Verification items for the finished model (mm, model axes). Face numbers are marked on the shaded views. Round coordinates to 2 decimals unless told otherwise and drop trailing zeros. Write each loop counter-clockwise with the first axis right and the second up, starting at its lowest first coordinate (ties: lowest second). Pieces come first, ordered by that corner, then holes. Notation, with made-up numbers: (3, -2) -> (31, -2) arc R12 cw to (31, 19) -> close; hole circle Ø8 at (66.25, 65). An arc over 180 degrees is marked (long way). Answer as a JSON object with one key per item and string values. Group by question number.
(1) Sectioned sample at A-A on x = 117.5. Record the cut outline in (y, z).
(2) Scan lines: L1, parallel to Y at x = 65, z = 8.55; L2, parallel to X at y = 44, z = 9.25; L3, parallel to Y at x = 113.5, z = 6.75. Record each from-to range of solid material in increasing order. Write a range as from..to.
(3) Gauge pin test, flat ends, axial feed: pin 1 Ø12 at (x, y) = (67, 18) entering from +Z; pin 2 Ø1.5 at (x, y) = (100.5, 12) entering from +Z. Record the tip position at first contact, or that the pin passes through.
(4) Draft check along Y on the marked faces 1, 2 and 3. Enter one of: released by +Y, released by -Y, zero draft, split by the parting line, or undercut.
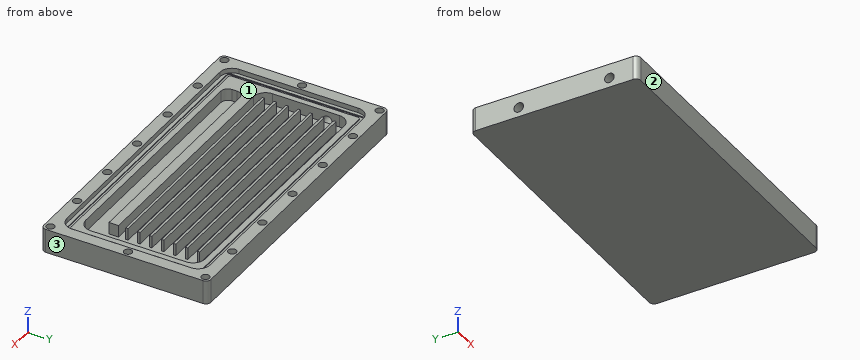
```python
from build123d import *

# Parameters (mm, degrees)
BOSS_EXTRU_1_DEPTH      = 10
ENL_V_MAT_EXTRU_1_DEPTH = 2
ENL_V_MAT_EXTRU_3_DEPTH = 5
ESQUISSE23_W            = 98
ESQUISSE23_H            = 1
BOSS_EXTRU_2_DEPTH      = 5
ENL_V_MAT_EXTRU_4_DEPTH = 0.4
ESQUISSE19_R            = 2
ENL_V_MAT_EXTRU_5_DEPTH = 10
D_GAGEMENT_M31_D        = 3.4
D_GAGEMENT_M31_DEPTH    = 3.978536948
D_GAGEMENT_M31_TIP      = 1.021463052


with BuildPart() as part:
    # Esquisse1 → Boss.-Extru.1 (new body)
    with BuildSketch(Plane.XY):
        with BuildLine():
            Line((2, 0), (128, 0))
            ThreePointArc((128, 0), (129.414213562, 0.585786438), (130, 2))
            Line((130, 2), (130, 68))
            ThreePointArc((130, 68), (129.414213562, 69.414213562), (128, 70))
            Line((128, 70), (2, 70))
            ThreePointArc((2, 70), (0.585786438, 69.414213562), (0, 68))
            Line((0, 68), (0, 2))
            ThreePointArc((0, 2), (0.585786438, 0.585786438), (2, 0))
        make_face()
    extrude(amount=BOSS_EXTRU_1_DEPTH)

    # Esquisse18 → Enlèv. mat.-Extru.1 (cut)
    with BuildSketch(Plane.XY.offset(10)):
        with BuildLine():
            Line((10, 5), (120, 5))
            ThreePointArc((120, 5), (123.535533906, 6.464466094), (125, 10))
            Line((125, 10), (125, 60))
            ThreePointArc((125, 60), (123.535533906, 63.535533906), (120, 65))
            Line((120, 65), (10, 65))
            ThreePointArc((10, 65), (6.464466094, 63.535533906), (5, 60))
            Line((5, 60), (5, 10))
            ThreePointArc((5, 10), (6.464466094, 6.464466094), (10, 5))
        make_face()
    extrude(amount=-ENL_V_MAT_EXTRU_1_DEPTH, mode=Mode.SUBTRACT)

    # Esquisse20 → Enlèv. mat.-Extru.3 (cut)
    with BuildSketch(Plane.XY.offset(8)):
        with BuildLine():
            Line((15, 60), (115, 60))
            ThreePointArc((115, 60), (118.535533906, 58.535533906), (120, 55))
            Line((120, 55), (120, 15))
            ThreePointArc((120, 15), (118.535533906, 11.464466094), (115, 10))
            Line((115, 10), (18, 10))
            ThreePointArc((18, 10), (15.878679656, 10.878679656), (15, 13))
            Line((15, 13), (15, 15))
            ThreePointArc((15, 15), (15.878679656, 17.121320344), (18, 18))
            Line((18, 18), (112, 18))
            Line((112, 18), (112, 22))
            Line((112, 22), (15, 22))
            ThreePointArc((15, 22), (11.464466094, 23.464466094), (10, 27))
            Line((10, 27), (10, 55))
            ThreePointArc((10, 55), (11.464466094, 58.535533906), (15, 60))
        make_face()
    extrude(amount=-ENL_V_MAT_EXTRU_3_DEPTH, mode=Mode.SUBTRACT)

    # Esquisse23 → Boss.-Extru.2 (add)
    with BuildSketch(Plane.XY.offset(3)):
        with Locations((62.966066354, 55.5)):
            Rectangle(ESQUISSE23_W, ESQUISSE23_H)
        with Locations((62.966066354, 50.5)):
            Rectangle(ESQUISSE23_W, ESQUISSE23_H)
        with Locations((62.966066354, 45.5)):
            Rectangle(ESQUISSE23_W, ESQUISSE23_H)
        with Locations((62.966066354, 40.5)):
            Rectangle(ESQUISSE23_W, ESQUISSE23_H)
        with Locations((62.966066354, 35.5)):
            Rectangle(ESQUISSE23_W, ESQUISSE23_H)
        with Locations((62.966066354, 30.5)):
            Rectangle(ESQUISSE23_W, ESQUISSE23_H)
        with Locations((62.966066354, 25.5)):
            Rectangle(ESQUISSE23_W, ESQUISSE23_H)
    extrude(amount=BOSS_EXTRU_2_DEPTH)

    # Esquisse24 → Enlèv. mat.-Extru.4 (cut)
    with BuildSketch(Plane.XY.offset(8)):
        with BuildLine():
            Line((6.5, 62.5), (6.5, 7.5))
            ThreePointArc((6.5, 7.5), (6.792893219, 6.792893219), (7.5, 6.5))
            Line((7.5, 6.5), (7.967348912, 6.5))
            Line((7.967348912, 6.5), (122.5, 6.5))
            ThreePointArc((122.5, 6.5), (123.207106781, 6.792893219), (123.5, 7.5))
            Line((123.5, 7.5), (123.5, 62.5))
            ThreePointArc((123.5, 62.5), (123.207106781, 63.207106781), (122.5, 63.5))
            Line((122.5, 63.5), (7.5, 63.5))
            ThreePointArc((7.5, 63.5), (6.792893219, 63.207106781), (6.5, 62.5))
        make_face()
        with BuildLine():
            Line((8.6, 62.4), (121.4, 62.4))
            ThreePointArc((121.4, 62.4), (122.107106781, 62.107106781), (122.4, 61.4))
            Line((122.4, 61.4), (122.4, 8.6))
            ThreePointArc((122.4, 8.6), (122.107106781, 7.892893219), (121.4, 7.6))
            Line((121.4, 7.6), (8.6, 7.6))
            ThreePointArc((8.6, 7.6), (7.892893219, 7.892893219), (7.6, 8.6))
            Line((7.6, 8.6), (7.6, 61.4))
            ThreePointArc((7.6, 61.4), (7.892893219, 62.107106781), (8.6, 62.4))
        make_face(mode=Mode.SUBTRACT)
    extrude(amount=-ENL_V_MAT_EXTRU_4_DEPTH, mode=Mode.SUBTRACT)

    # Esquisse19 → Enlèv. mat.-Extru.5 (cut)
    with BuildSketch(Plane.ZY):
        with Locations((4, 50)):
            Circle(ESQUISSE19_R)
        with Locations((4, 12)):
            Circle(ESQUISSE19_R)
    extrude(amount=-ENL_V_MAT_EXTRU_5_DEPTH, mode=Mode.SUBTRACT)

    # Dégagement M31
    with Locations(Plane.XY.offset(10)):
        with Locations((127.5, 67.5), (108.32, 67.5), (86.66, 67.5), (65, 67.5), (43.34, 67.5), (21.68, 67.5), (2.5, 67.5), (2.5, 35), (2.5, 2.5), (21.68, 2.5), (43.34, 2.5), (65.266790711, 2.5), (86.66, 2.5), (108.32, 2.5), (127.5, 2.5), (127.5, 35)):
            Hole(D_GAGEMENT_M31_D / 2, depth=D_GAGEMENT_M31_DEPTH)
            with Locations((0, 0, -(D_GAGEMENT_M31_DEPTH + D_GAGEMENT_M31_TIP / 2))):  # 118° drill point
                Cone(0, D_GAGEMENT_M31_D / 2, D_GAGEMENT_M31_TIP, mode=Mode.SUBTRACT)


solid = part.part
```
Computed values:
{
 "1": {"outline": "(0, 0) -> (70, 0) -> (70, 10) -> (65, 10) -> (65, 8) -> (63.5, 8) -> (63.5, 7.6) -> (62.4, 7.6) -> (62.4, 8) -> (59.33, 8) -> (59.33, 3) -> (10.67, 3) -> (10.67, 8) -> (7.6, 8) -> (7.6, 7.6) -> (6.5, 7.6) -> (6.5, 8) -> (5, 8) -> (5, 10) -> (0, 10) -> close"},
 "2": {"L1": "0..0.82, 4.18..5, 65..65.8, 69.2..70", "L2": "0..5, 125..130", "L3": "0..10, 60..70"},
 "3": {"pin 1": "z = 8", "pin 2": "z = 3"},
 "4": {"face 1": "undercut", "face 2": "released by -Y", "face 3": "zero draft"}
}
